```python
from build123d import *

# Parameters (mm, degrees)
F0_R         = 15
F0_R_2       = 0.5
F0_R_3       = 0.85
F1_DEPTH     = 0.762
F3_DEPTH     = 0.262
F4_R         = 4.05
F5_DEPTH     = 0.5
F6_T4_DEPTH  = 0.6914880487
F6_T9_DEPTH  = 0.6914880487
F6_T11_DEPTH = 0.3832692911
F6_T13_DEPTH = 0.4252513356
F7_R         = 0.3
F8_DEPTH     = 0.3


# Not quite as in the source:
# - a fillet or chamfer that OpenCascade refuses, or shapes differently, is made with other operations: its cross-section is extruded or revolved along the edge and cut away or added


with BuildPart() as f1:
    # F0 (on Top) → F1 (new body)
    with BuildSketch(Plane.XY):
        Circle(F0_R)
        with BuildLine():
            ThreePointArc((-3.7629684096, -5.4024791326), (-2.2734929609, -3.548324336), (0, -2.85))
            ThreePointArc((0, -2.85), (2.2734929609, -3.548324336), (3.7629684096, -5.4024791326))
            ThreePointArc((3.7629684096, -5.4024791326), (3.6929780242, -5.6394712752), (3.4461538031, -5.6275660849))
            ThreePointArc((3.4461538031, -5.6275660849), (1.9616904878, -5.2330123256), (0.7378557396, -6.1612000827))
            ThreePointArc((0.7378557396, -6.1612000827), (0.6097380289, -6.2645935657), (0.4474599736, -6.2368412165))
            ThreePointArc((0.4474599736, -6.2368412165), (0.233958301, -6.1349748283), (0, -6.1))
            ThreePointArc((0, -6.1), (-0.233958301, -6.1349748283), (-0.4474599736, -6.2368412165))
            ThreePointArc((-0.4474599736, -6.2368412165), (-0.6097380289, -6.2645935657), (-0.7378557396, -6.1612000827))
            ThreePointArc((-0.7378557396, -6.1612000827), (-1.9616904878, -5.2330123256), (-3.4461538031, -5.6275660849))
            ThreePointArc((-3.4461538031, -5.6275660849), (-3.6929780242, -5.6394712752), (-3.7629684096, -5.4024791326))
        make_face(mode=Mode.SUBTRACT)
        with Locations((-6.7, 0)):
            Circle(F0_R_2, mode=Mode.SUBTRACT)
        Circle(F0_R_3, mode=Mode.SUBTRACT)
        with Locations((6.7, 0)):
            Circle(F0_R_2, mode=Mode.SUBTRACT)
        with Locations((0, 7.2)):
            Circle(F0_R_2, mode=Mode.SUBTRACT)
    extrude(amount=F1_DEPTH)

    # F2 (on face) → F3 (cut)
    with BuildSketch(Plane.XY.offset(0.762)):
        with BuildLine():
            ThreePointArc((4, -8.8543774485), (4.0930955032, -9.0234082994), (4.2857142857, -9.0350790291))
            ThreePointArc((4.2857142857, -9.0350790291), (0, 10), (-4.2857142857, -9.0350790291))
            ThreePointArc((-4.2857142857, -9.0350790291), (-4.0930955032, -9.0234082994), (-4, -8.8543774485))
            Line((-4, -8.8543774485), (-4, -8.2))
            ThreePointArc((-4, -8.2), (-3.9414213562, -8.0585786438), (-3.8, -8))
            Line((-3.8, -8), (0, -8))
            Line((0, -8), (3.8, -8))
            ThreePointArc((3.8, -8), (3.9414213562, -8.0585786438), (4, -8.2))
            Line((4, -8.2), (4, -8.8543774485))
        make_face()
    extrude(amount=-F3_DEPTH, mode=Mode.SUBTRACT)

    # F4 (on face) → F5 (cut)
    with BuildSketch(Plane.XY.offset(0.762)):
        with Locations((0, 7.2)):
            Circle(F4_R)
        with Locations((6.7, 0)):
            Circle(F4_R)
        with Locations((-6.7, 0)):
            Circle(F4_R)
        with BuildLine():
            ThreePointArc((3.8, -8), (3.8470411203, -8.0056108722), (3.8914428234, -8.02212867))
            ThreePointArc((3.8914428234, -8.02212867), (0, -2.85), (-3.8914428234, -8.02212867))
            ThreePointArc((-3.8914428234, -8.02212867), (-3.8470411203, -8.0056108722), (-3.8, -8))
            Line((-3.8, -8), (3.8, -8))
        make_face()
    extrude(amount=-F5_DEPTH, mode=Mode.SUBTRACT)

    # F6: fillet of radius 0.2 on 8 edges, made by hand


with BuildPart() as f6_tool2:
    # F6_s3 → F6_t4 (new body)
    with BuildSketch(Plane.XY.offset(0.5)):
        with BuildLine():
            ThreePointArc((3.9377859629, -7.8467532468), (3.8671202695, -7.9570838142), (3.7433273968, -8))
            Line((3.7433273968, -8), (3.7433273968, -8.02))
            ThreePointArc((3.7433273968, -8.02), (3.8, -8.02), (3.8822985411, -8.039915803))
            Line((3.8822985411, -8.039915803), (3.910659825, -8.0276700461))
            ThreePointArc((3.910659825, -8.0276700461), (3.9349326547, -7.9398100803), (3.9572318195, -7.8514285714))
            Line((3.9572318195, -7.8514285714), (3.9377859629, -7.8467532468))
        make_face()
    extrude(amount=-F6_T4_DEPTH)

    split(bisect_by=Plane.XY, keep=Keep.TOP)


with BuildPart() as f1_1:
    add(f1.part)

    # F6_t1: union F6_tool2
    add(f6_tool2.part)


with BuildPart() as f6_tool7:
    # F6_s8 → F6_t9 (new body)
    with BuildSketch(Plane.XY.offset(0.5)):
        with BuildLine():
            ThreePointArc((-3.9377859629, -7.8467532468), (-3.8671202695, -7.9570838142), (-3.7433273968, -8))
            Line((-3.7433273968, -8), (-3.7433273968, -8.02))
            ThreePointArc((-3.7433273968, -8.02), (-3.8, -8.02), (-3.8822985411, -8.039915803))
            Line((-3.8822985411, -8.039915803), (-3.910659825, -8.0276700461))
            ThreePointArc((-3.910659825, -8.0276700461), (-3.9349326547, -7.9398100803), (-3.9572318195, -7.8514285714))
            Line((-3.9572318195, -7.8514285714), (-3.9377859629, -7.8467532468))
        make_face()
    extrude(amount=-F6_T9_DEPTH)

    split(bisect_by=Plane.XY, keep=Keep.TOP)


with BuildPart() as f1_2:
    add(f1_1.part)

    # F6_t6: union F6_tool7
    add(f6_tool7.part)

    # F6_s12 → F6_t11 (cut)
    with BuildSketch(Plane.XY.offset(0.5)):
        with BuildLine():
            ThreePointArc((-9.5747366111, 2.8852068953), (-9.5935467273, 2.8420149313), (-9.6219381036, 2.8044211022))
            ThreePointArc((-9.6219381036, 2.8044211022), (-9.6053293925, 2.8216238447), (-9.588619403, 2.8387282266))
            ThreePointArc((-9.588619403, 2.8387282266), (-9.5817061892, 2.8619759788), (-9.5747366111, 2.8852068953))
        make_face()
        with BuildLine():
            ThreePointArc((-9.6219381036, -2.8044211022), (-9.5935467273, -2.8420149313), (-9.5747366111, -2.8852068953))
            ThreePointArc((-9.5747366111, -2.8852068953), (-9.5817061892, -2.8619759788), (-9.588619403, -2.8387282266))
            ThreePointArc((-9.588619403, -2.8387282266), (-9.6053293925, -2.8216238447), (-9.6219381036, -2.8044211022))
        make_face()
        with BuildLine():
            ThreePointArc((9.6219381036, 2.8044211022), (9.5935467273, 2.8420149313), (9.5747366111, 2.8852068953))
            ThreePointArc((9.5747366111, 2.8852068953), (9.5817061892, 2.8619759788), (9.588619403, 2.8387282266))
            ThreePointArc((9.588619403, 2.8387282266), (9.6053293925, 2.8216238447), (9.6219381036, 2.8044211022))
        make_face()
        with BuildLine():
            ThreePointArc((9.6219381036, -2.8044211022), (9.5935467273, -2.8420149313), (9.5747366111, -2.8852068953))
            ThreePointArc((9.5747366111, -2.8852068953), (9.5817061892, -2.8619759788), (9.588619403, -2.8387282266))
            ThreePointArc((9.588619403, -2.8387282266), (9.6053293925, -2.8216238447), (9.6219381036, -2.8044211022))
        make_face()
    extrude(amount=F6_T11_DEPTH, mode=Mode.SUBTRACT)

    # F6_s14 → F6_t13 (cut)
    with BuildSketch(Plane.XY.offset(0.5)):
        with BuildLine():
            ThreePointArc((3.4582244159, 9.3829997277), (3.4038059187, 9.4134107296), (3.3613941322, 9.4590992647))
            ThreePointArc((3.3613941322, 9.4590992647), (3.3792435663, 9.4323111163), (3.3968795208, 9.4053819444))
            ThreePointArc((3.3968795208, 9.4053819444), (3.427570238, 9.3942409094), (3.4582244159, 9.3829997277))
        make_face()
        with BuildLine():
            ThreePointArc((-3.3613941322, 9.4590992647), (-3.4038059187, 9.4134107296), (-3.4582244159, 9.3829997277))
            ThreePointArc((-3.4582244159, 9.3829997277), (-3.427570238, 9.3942409094), (-3.3968795208, 9.4053819444))
            ThreePointArc((-3.3968795208, 9.4053819444), (-3.3792435663, 9.4323111163), (-3.3613941322, 9.4590992647))
        make_face()
    extrude(amount=F6_T13_DEPTH, mode=Mode.SUBTRACT)

    # F7 (on face) → F8 (cut)
    with BuildSketch(Plane(origin=(0, 0, 0), x_dir=(1, 0, 0), z_dir=(0, 0, -1))):
        with Locations((8.42, -7.15)):
            Circle(F7_R)
        with Locations((-8.42, 7.15)):
            Circle(F7_R)
    extrude(amount=-F8_DEPTH, mode=Mode.SUBTRACT)


solid = f1_2.part
```
CAD build for the part. Positions are in the model's coordinates, mm. A direction names the side the tool comes from. Give positions to 0.01 mm unless a question says otherwise; leave off trailing zeros. Order: outer loops, then holes, each group sorted by start corner. A loop starts at its lowest first (then second) coordinate and runs counter-clockwise, first axis right, second up. Notation, with made-up numbers: M 59,26.25 L 118,26.25 A9 cw 118,38.25 Z; hole C 71.25,-19.75 d11. An arc over 180 degrees is marked long. Put each result on its own line as item: value. Start each with the question number.
(1) Drill centre lines: line 1 along X through (y, z) = (7.15, 0.1); line 2 along Z through (x, y) = (-6.75, 7); line 3 along Y through (x, z) = (-1.75, 0.45). Where is each one in solid material? Low to high.
(2) Saw through at A-A, the plane y = 0. Write the cut outline in (x, z).
(3) Saw through at B-B, the plane x = -6.7. Write the cut outline in (y, z).
(4) Which spindle directions (+Z, -Z, +X, -X, +Y, -Y) get a long thin tool onto all of the face, cutting with end or side? Do faces 1 (the cylindrical face through (-14.985, 0.66, 0.376)), 2 (the cylindrical face through (-0.527, 11.216, 0.46)). Say none if no direction does.
(5) Saw through at C-C, the plane y = 8.25. Write the cut outline in (x, z), then the cut area to 3 significant figures.
(6) Saw through at D-D, the plane y = -11. Write the cut outline in (x, z), then the cut area to 3 significant figures.
(7) Flat gauge pins, fed straight in: pin 1 Ø2 at (x, y) = (0, 0) entering from +Z; pin 2 Ø2 at (x, y) = (0.5, -6.5) entering from +Z. Where does each tip first touch, or does it go through?
Check result:
1. line 1: x = -13.19 to -0.5, 0.5 to 8.12, 8.72 to 13.19
1. line 2: z = 0 to 0.5
1. line 3: y = -14.9 to -8, -3.25 to 3.55, 10.85 to 14.9
2. outline: M -15,0 L -7.2,0 L -7.2,0.26 L -10.75,0.26 L -10.75,0.76 L -15,0.76 Z; M -6.2,0 L -0.85,0 L -0.85,0.5 L -2.65,0.5 L -2.65,0.26 L -6.2,0.26 Z; M 0.85,0 L 6.2,0 L 6.2,0.26 L 2.65,0.26 L 2.65,0.5 L 0.85,0.5 Z; M 7.2,0 L 15,0 L 15,0.76 L 10.75,0.76 L 10.75,0.26 L 7.2,0.26 Z
3. outline: M -13.42,0 L -0.5,0 L -0.5,0.26 L -4.05,0.26 L -4.05,0.5 L -7.42,0.5 L -7.42,0.76 L -13.42,0.76 Z; M 0.5,0 L 13.42,0 L 13.42,0.76 L 7.42,0.76 L 7.42,0.5 L 4.05,0.5 L 4.05,0.26 L 0.5,0.26 Z
4. face 1: +Z, -Z
4. face 2: +Z
5. outline: M -12.53,0 L 12.53,0 L 12.53,0.76 L 5.65,0.76 L 5.65,0.5 L 3.91,0.5 L 3.91,0.26 L -3.91,0.26 L -3.91,0.5 L -5.65,0.5 L -5.65,0.76 L -12.53,0.76 Z
5. area: 14.3 mm2
6. outline: M -10.2,0 L 10.2,0 L 10.2,0.76 L -10.2,0.76 Z
6. area: 15.5 mm2
7. pin 1: stops at z = 0.5
7. pin 2: stops at z = 0.26
